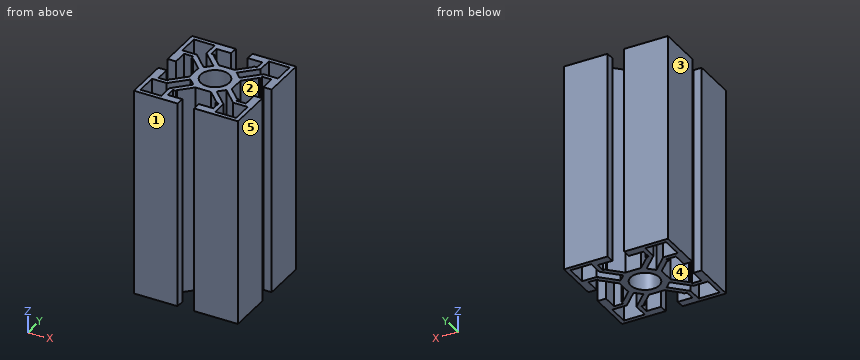
from build123d import *

# Parameters (mm, degrees)
SKETCH_A01_1_R     = 6.85
SKETCH_A01_1_W     = 10
SKETCH_A01_1_H     = 10
EXTRUDE1_DEPTH     = 100
CUT_EXTRUDE1_DEPTH = 101
CIRPATTERN1_COUNT  = 4


with BuildPart() as part:
    # Sketch A01-1 → Extrude1 (new body)
    with BuildSketch(Plane.XY):
        Polygon((-16.5, -11), (-16.5, -9.5), (-15.863961, -9.5), (-10.14602885, -3.78206785), (-10.14602885, 3.78206785), (-15.863961, 9.5), (-16.5, 9.5), (-16.5, 11), (-21, 11), (-21, 4), (-25, 4), (-25, 25), (-4, 25), (-4, 21), (-11, 21), (-11, 16.5), (-9.5, 16.5), (-9.5, 15.863961), (-3.78206785, 10.14602885), (3.78206785, 10.14602885), (9.5, 15.863961), (9.5, 16.5), (11, 16.5), (11, 21), (4, 21), (4, 25), (25, 25), (25, 4), (21, 4), (21, 11), (16.5, 11), (16.5, 9.5), (15.863961, 9.5), (10.14602885, 3.78206785), (10.14602885, -3.78206785), (15.863961, -9.5), (16.5, -9.5), (16.5, -11), (21, -11), (21, -4), (25, -4), (25, -25), (4, -25), (4, -21), (11, -21), (11, -16.5), (9.5, -16.5), (9.5, -15.863961), (3.78206785, -10.14602885), (-3.78206785, -10.14602885), (-9.5, -15.863961), (-9.5, -16.5), (-11, -16.5), (-11, -21), (-4, -21), (-4, -25), (-25, -25), (-25, -4), (-21, -4), (-21, -11), align=None)
        Circle(SKETCH_A01_1_R, mode=Mode.SUBTRACT)
        with Locations((-18, -18)):
            Rectangle(SKETCH_A01_1_W, SKETCH_A01_1_H, mode=Mode.SUBTRACT)
        with Locations((18, -18)):
            Rectangle(SKETCH_A01_1_W, SKETCH_A01_1_H, mode=Mode.SUBTRACT)
        with Locations((-18, 18)):
            Rectangle(SKETCH_A01_1_W, SKETCH_A01_1_H, mode=Mode.SUBTRACT)
        with Locations((18, 18)):
            Rectangle(SKETCH_A01_1_W, SKETCH_A01_1_H, mode=Mode.SUBTRACT)
    extrude(amount=-EXTRUDE1_DEPTH)

    # Sketch1 → Cut-Extrude1 (cut, through all)
    with BuildSketch(Plane.XY):
        Polygon((-15.993494496, 13), (-8.602622103, 5.609127607), (-5.609127607, 8.602622103), (-13, 15.993494496), align=None)
    cut_extrude1 = extrude(amount=-CUT_EXTRUDE1_DEPTH, mode=Mode.SUBTRACT)

    # CirPattern1: Cut-Extrude1 ×4 about axis
    cirpattern1_axis = Axis((0, 0, 0), (0, 0, 1))
    for i in range(1, CIRPATTERN1_COUNT):
        add(cut_extrude1.rotate(cirpattern1_axis, i * 360 / CIRPATTERN1_COUNT), mode=Mode.SUBTRACT)


solid = part.part
CAD build for the part. Positions are in the model's coordinates, mm. Face numbers are marked on the shaded views. A direction names the side the tool comes from. Round coordinates to 2 decimals unless told otherwise and drop trailing zeros. Write each loop counter-clockwise with the first axis right and the second up, starting at its lowest first coordinate (ties: lowest second). Pieces come first, ordered by that corner, then holes. Notation, with made-up numbers: M -29.5,30.25 L 10.5,30.25 A34 ccw 10.5,64.25 Z; hole C 60.25,12 d4. An arc over 180 degrees is marked long. Put each result on its own line as item: value. Start each with the question number.
1) Saw through at B-B, the plane x = 19.5. Write the cut outline in (y, z), and give its area (3 significant figures).
2) Saw through at A-A, the plane x = 0. Write the cut outline in (y, z), and give its area (3 significant figures).
3) Saw through at D-D, the plane z = -54.5. Count the separate pieces of the cut face and the enclosed holes in it, and give its area (3 significant figures).
4) Drill centre lines: probe 1 along Y at (x, z) = (20, -50); probe 2 along X at (y, z) = (22, -91). Where is each one in solid material? Low to high. Write a range as [from, to].
5) 3-axis set-ups, long thin cutter, end or side, ignore diameter. For the marked faces 4 and 5: which of +Z, -Z, +X, -X, +Y, -Y reach the whole face in a straight line?
6) Pin check, flat tip, straight feed: pin 1 Ø4 at (y, z) = (-1.5, -31) entering from +X. Stop position of the tip, or through.
7) Pull direction Y, two halves, no side cores. Call the marked faces 1, 2 and 3: pulls with the +Y half, pulls with the -Y half, needs draft (parallel to the pull), parting line crosses it, or undercut.
Resolved:
1. outline: M -25,-100 L -23,-100 L -23,0 L -25,0 Z; M -13,-100 L -11,-100 L -11,0 L -13,0 Z; M 11,-100 L 13,-100 L 13,0 L 11,0 Z; M 23,-100 L 25,-100 L 25,0 L 23,0 Z
1. area: 800 mm²
2. outline: M -10.15,-100 L -6.85,-100 L -6.85,0 L -10.15,0 Z; M 6.85,-100 L 10.15,-100 L 10.15,0 L 6.85,0 Z
2. area: 659 mm²
3. separate pieces: 1
3. enclosed holes: 5
3. area: 917 mm²
4. probe 1: [-25, -23], [-13, -11], [11, 13], [23, 25]
4. probe 2: [-25, -23], [-13, -4], [4, 13], [23, 25]
5. face 4: +Z, -Z
5. face 5: +Z, -Z, +X, +Y, -Y
6. pin 1: x = 10.15
7. face 1: pulls with the -Y half
7. face 2: undercut
7. face 3: needs draft
